from build123d import *

# Parameters (mm, degrees)
SKETCH1_W                 = 114.3
SKETCH1_H                 = 177.8
SKETCH1_W_2               = 101.6
SKETCH1_H_2               = 165.1
BOSS_EXTRUDE1_DEPTH       = 4.7625
SKETCH2_W                 = 12.38677804
SKETCH2_H                 = 4.7625
SKETCH2_W_2               = 12.7
BOSS_EXTRUDE2_DEPTH       = 4.7625
SKETCH3_W                 = 12.7
SKETCH3_H                 = 4.7625
BOSS_EXTRUDE3_DEPTH       = 4.7625
FILLET1_R                 = 2.54
SKETCH4_W                 = 114.3
SKETCH4_H                 = 12.7
BOSS_EXTRUDE4_DEPTH       = 4.7625
F_6_CLEARANCE_HOLE1_D     = 3.7973
F_6_CLEARANCE_HOLE1_DEPTH = 25.4
F_6_CLEARANCE_HOLE1_TIP   = 1.140824014


with BuildPart() as part:
    # Sketch1 → Boss-Extrude1 (new body)
    with BuildSketch(Plane(origin=(0, 0, 0), x_dir=(1, 0, 0), z_dir=(0, 1, 0))):
        Rectangle(SKETCH1_W, SKETCH1_H)
        Rectangle(SKETCH1_W_2, SKETCH1_H_2, mode=Mode.SUBTRACT)
    extrude(amount=BOSS_EXTRUDE1_DEPTH)

    # Sketch2 → Boss-Extrude2 (add)
    with BuildSketch(Plane.XY.offset(88.9)):
        with Locations((-38.1, 2.38125)):
            Rectangle(SKETCH2_W, SKETCH2_H)
        with Locations((12.7, 2.38125)):
            Rectangle(SKETCH2_W_2, SKETCH2_H)
    extrude(amount=BOSS_EXTRUDE2_DEPTH)

    # Sketch3 → Boss-Extrude3 (add)
    with BuildSketch(Plane(origin=(0, 0, -88.9), x_dir=(-1, 0, 0), z_dir=(0, 0, -1))):
        with Locations((-38.1, 2.38125)):
            Rectangle(SKETCH3_W, SKETCH3_H)
        with Locations((12.7, 2.38125)):
            Rectangle(SKETCH3_W, SKETCH3_H)
    extrude(amount=BOSS_EXTRUDE3_DEPTH)

    # Fillet1
    fillet1_edges = [part.edges().sort_by_distance(p)[0] for p in [
        (50.8, 2.38125, 82.55),
        (50.8, 2.38125, -82.55),
        (-50.8, 2.38125, -82.55),
        (-50.8, 2.38125, 82.55),
    ]]
    fillet(fillet1_edges, radius=FILLET1_R)

    # Sketch4 → Boss-Extrude4 (add)
    with BuildSketch(Plane(origin=(0, 4.7625, 0), x_dir=(1, 0, 0), z_dir=(0, 1, 0))):
        Rectangle(SKETCH4_W, SKETCH4_H)
    extrude(amount=-BOSS_EXTRUDE4_DEPTH)

    # #6 Clearance Hole1
    with Locations(Plane(origin=(0, 4.7625, 0), x_dir=(-1, 0, 0), z_dir=(0, 1, 0))):
        with Locations((31.75, 0), (-31.75, 0)):
            Hole(F_6_CLEARANCE_HOLE1_D / 2, depth=F_6_CLEARANCE_HOLE1_DEPTH)
            with Locations((0, 0, -(F_6_CLEARANCE_HOLE1_DEPTH + F_6_CLEARANCE_HOLE1_TIP / 2))):  # 118° drill point
                Cone(0, F_6_CLEARANCE_HOLE1_D / 2, F_6_CLEARANCE_HOLE1_TIP, mode=Mode.SUBTRACT)


solid = part.part
Model file for the job. Use its own axes, mm. A direction names the side the tool comes from. Give positions to 0.01 mm unless a question says otherwise; leave off trailing zeros. Write each loop counter-clockwise with the first axis right and the second up, starting at its lowest first coordinate (ties: lowest second). Pieces come first, ordered by that corner, then holes. Notation, with made-up numbers: M 34,28.5 L 40,28.5 A22 cw 40,58.5 Z; hole C 34,71.5 d1. An arc over 180 degrees is marked long. One line per item, written item: value. Start each with the question number.
Q1. Saw through at A-A, the plane z = 0. Write the cut outline in (x, y), plus the area to 3 significant figures.
Q2. Saw through at D-D, the plane z = -53.5. Write the cut outline in (x, y), plus the area to 3 significant figures.
Q3. Drop flat-ended pins along their axis: pin 1 Ø2.5 at (x, y) = (-21, 1.5) entering from +Z; pin 2 Ø2.5 at (x, y) = (24, 3) entering from -Z; pin 3 Ø2.5 at (y, z) = (3, 92.5) entering from -X. Give the stop position or say it passes through.
Q4. Saw through at B-B, the plane y = 3.9. State how many separate pieces and enclosed holes the cut face has, plus the area to 3 significant figures.
Q5. Saw through at C-C, the plane x = 13. Write the cut outline in (y, z), plus the area to 3 significant figures.
Q6. 3-axis set-ups, long thin cutter, end or side, ignore diameter. For faces 1 (the flat face through (-31.907, 2, 91)), 2 (the flat face through (-19.05, 2, -91)), 3 (the flat face through (12, 2, -88.9)), 4 (the flat face through (-1, 2, 6.35)), 5 (the flat face through (38, 2, 88.9)): which of +Z, -Z, +X, -X, +Y, -Y reach the whole face in a straight line?
Q7. Two-plate mould, pull along X, no slides. Class faces 6 (the flat face through (6.35, 2, 91)), 7 (the flat face through (-57.15, 2, 1)), 8 (the flat face through (-51, 2, 88.9)), 9 (the flat face through (-13, 2, 88.9)): +X half, -X half, draft (parallel to the pull), parting line (faces both ways), or undercut.
Q8. Probe probe 1 along Z at (x, y) = (-5, 1.1); probe 2 along Z at (x, y) = (-31.75, 1.45); probe 3 along Z at (x, y) = (-42.5, 3.05). List the from-to ranges inside material, lowest first. Write a range as [from, to].
Output values:
1. outline: M -57.15,0 L -33.65,0 L -33.65,4.76 L -57.15,4.76 Z; M -29.85,0 L 29.85,0 L 29.85,4.76 L -29.85,4.76 Z; M 33.65,0 L 57.15,0 L 57.15,4.76 L 33.65,4.76 Z
1. area: 508 mm²
2. outline: M -57.15,0 L -50.8,0 L -50.8,4.76 L -57.15,4.76 Z; M 50.8,0 L 57.15,0 L 57.15,4.76 L 50.8,4.76 Z
2. area: 60.5 mm²
3. pin 1: stops at z = 88.9
3. pin 2: stops at z = -88.9
3. pin 3: stops at x = -44.29
4. separate pieces: 1
4. enclosed holes: 4
4. area: 5,060 mm²
5. outline: M 0,-88.9 L 4.76,-88.9 L 4.76,-82.55 L 0,-82.55 Z; M 0,-6.35 L 4.76,-6.35 L 4.76,6.35 L 0,6.35 Z; M 0,82.55 L 4.76,82.55 L 4.76,93.66 L 0,93.66 Z
5. area: 144 mm²
6. face 1: +Z, +Y, -Y
6. face 2: -Z, -X, +Y, -Y
6. face 3: -Z, +Y, -Y
6. face 4: +Y, -Y
6. face 5: +Z, +X, +Y, -Y
7. face 6: undercut
7. face 7: -X half
7. face 8: draft
7. face 9: undercut
8. probe 1: z = [-88.9, -82.55], [-6.35, 6.35], [82.55, 88.9]
8. probe 2: z = [-88.9, -82.55], [-6.35, -1.9], [1.9, 6.35], [82.55, 88.9]
8. probe 3: z = [-88.9, -82.55], [-6.35, 6.35], [82.55, 93.66]
